from build123d import *

# Parameters (mm, degrees)
F1_W     = 54.708
F1_H     = 77.4
F2_DEPTH = 1.5
F3_W     = 8.434
F3_H     = 27.322
F3_R     = 1.4
F3_R_2   = 1
F3_R_3   = 2.25
F4_DEPTH = 1.501
F5_R     = 4
F6_R     = 3
F6_R_2   = 1
F7_DEPTH = 4
F9_R     = 3


# Not quite as in the source:
# - a fillet or chamfer that OpenCascade refuses, or shapes differently, is made with other operations: its cross-section is extruded or revolved along the edge and cut away or added


with BuildPart() as f2:
    # F1 (on face) → F2 (new body)
    with BuildSketch(Plane.XY):
        with Locations((25.654, 37)):
            Rectangle(F1_W, F1_H)
    extrude(amount=F2_DEPTH)

    # F3 (on face) → F4 (cut, through all)
    with BuildSketch(Plane.XY.offset(1.5)):
        Polygon((44.574, 16.81), (6.734, 16.81), (-1.7, 16.81), (-1.7, -1.7), (53.008, -1.7), (53.008, 16.81), align=None)
        with Locations((2.517, 38.905)):
            Rectangle(F3_W, F3_H)
        with Locations((48.791, 38.905)):
            Rectangle(F3_W, F3_H)
        Polygon((-1.7, 61), (6.734, 61), (44.574, 61), (53.008, 61), (53.008, 75.7), (-1.7, 75.7), align=None)
        with Locations((2.517, 21.027)):
            Circle(F3_R)
        with Locations((48.791, 21.027)):
            Circle(F3_R)
        with Locations((48.791, 56.783)):
            Circle(F3_R)
        with Locations((2.517, 56.783)):
            Circle(F3_R)
        with Locations((33.254, 53.605)):
            Circle(F3_R_2)
        with Locations((18.054, 24.205)):
            Circle(F3_R_2)
        with Locations((11.334, 42.75)):
            Circle(F3_R_3)
    extrude(amount=-F4_DEPTH, mode=Mode.SUBTRACT)

    # F5
    f5_edges = [f2.edges().sort_by_distance(p)[0] for p in [
        (-1.7, 61, 0.75),
        (-1.7, 52.566, 0.75),
        (-1.7, 25.244, 0.75),
        (-1.7, 16.81, 0.75),
        (6.734, 25.244, 0.75),
        (6.734, 52.566, 0.75),
        (53.008, 61, 0.75),
        (53.008, 52.566, 0.75),
        (44.574, 52.566, 0.75),
        (44.574, 25.244, 0.75),
        (53.008, 25.244, 0.75),
        (53.008, 16.81, 0.75),
    ]]
    fillet(f5_edges, radius=F5_R)

    # F6 (on face) → F7 (join)
    with BuildSketch(Plane.XY.offset(1.5)):
        with Locations((18.054, 24.205)):
            Circle(F6_R)
        with Locations((18.054, 24.205)):
            Circle(F6_R_2, mode=Mode.SUBTRACT)
        with Locations((33.254, 53.605)):
            Circle(F6_R)
        with Locations((33.254, 53.605)):
            Circle(F6_R_2, mode=Mode.SUBTRACT)
    extrude(amount=F7_DEPTH)

    # F8: chamfer of 0.5 x 5.7150261514 on 2 edges, made by hand


with BuildPart() as f8_tool2:
    # F8_s3 → F8_t4 (revolve)
    with BuildSketch(Plane.XZ.offset(-24.205)):
        Polygon((21.054, -0.2150261514), (20.554, 5.5), (21.054, 5.5), align=None)
    revolve(axis=Axis((18.054, 24.205, 5.5), (0, 0, 1)))

    split(bisect_by=Plane.XY.offset(1.5), keep=Keep.TOP)


with BuildPart() as f2_1:
    add(f2.part)

    # F8_t1: cut F8_tool2
    add(f8_tool2.part, mode=Mode.SUBTRACT)


with BuildPart() as f8_tool7:
    # F8_s8 → F8_t9 (revolve)
    with BuildSketch(Plane.XZ.offset(-53.605)):
        Polygon((36.254, -0.2150261514), (35.754, 5.5), (36.254, 5.5), align=None)
    revolve(axis=Axis((33.254, 53.605, 5.5), (0, 0, 1)))

    split(bisect_by=Plane.XY.offset(1.5), keep=Keep.TOP)


with BuildPart() as f2_2:
    add(f2_1.part)

    # F8_t6: cut F8_tool7
    add(f8_tool7.part, mode=Mode.SUBTRACT)

    # F9
    f9_edges = [f2_2.edges().sort_by_distance(p)[0] for p in [
        (15.204045, 24.205, 1.5),
        (30.404045, 53.605, 1.5),
    ]]
    fillet(f9_edges, radius=F9_R)


solid = f2_2.part
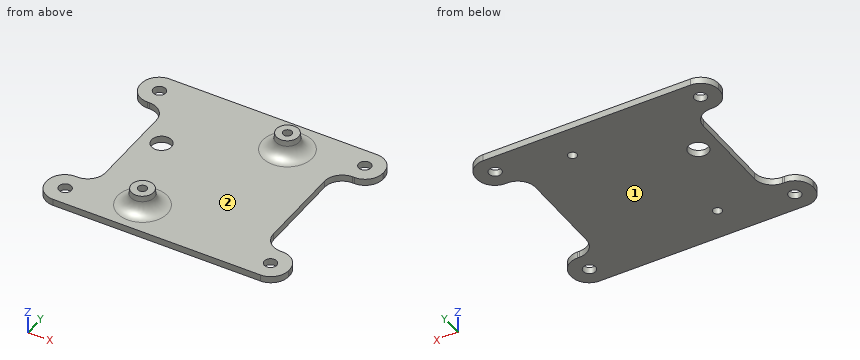
Design review of the part built by this model. Coordinates are the model's own, in mm. Face numbers are marked on the shaded views. A direction names the side the tool comes from. Coordinates: 2 decimals unless noted, no trailing zeros. Order: outer loops, then holes, each group sorted by start corner. A loop starts at its lowest first (then second) coordinate and runs counter-clockwise, first axis right, second up.
Item 1: For line 1 (Z direction, x = 2, y = 58.5); line 2 (X direction, y = 22, z = 0.75); line 3 (X direction, y = 54.5, z = 2.05), list the stretches that pass through material, from the lowest coordinate up.
Item 2: For the marked faces 1 and 2, list the 3-axis set-ups (+Z, -Z, +X, -X, +Y, -Y) from which the entire face can be reached by the end or side of a thin tool; tool diameter is ignored.
Item 3: Take a section at B-B, the plane z = 2.95. Write out the cut boundary in (x, y) (3 decimals).
Item 4: Take a section at A-A, the plane y = 42.75. Write out the cut boundary in (x, z).
Item 5: Take a section at C-C, the plane y = 31. Write out the cut boundary in (x, z).
Item 6: For pin 1 Ø3 at (x, y) = (48.791, 21.027) entering from +Z; pin 2 Ø1.6 at (y, z) = (41.5, 1) entering from +X, all flat-tipped, find the tip position at first contact; note any pin that passes through.
The answers:
1. line 1: z = 0 to 1.5
1. line 2: x = -1.63 to 1.51, 3.52 to 47.78, 49.8 to 52.94
1. line 3: x = 29.49 to 32.81, 33.7 to 37.02
2. face 1: -Z, +X, -X, +Y, -Y
2. face 2: +Z
3. outline: circle Ø6.061 at (18.054, 24.205); circle Ø6.061 at (33.254, 53.605); hole circle Ø2 at (18.054, 24.205); hole circle Ø2 at (33.254, 53.605)
4. outline: (6.73, 0) - (9.08, 0) - (9.08, 1.5) - (6.73, 1.5) - close; (13.58, 0) - (44.57, 0) - (44.57, 1.5) - (13.58, 1.5) - close
5. outline: (6.73, 0) - (44.57, 0) - (44.57, 1.5) - (6.73, 1.5) - close
6. pin 1: stops at z = 1.5
6. pin 2: stops at x = 44.57
